Input: dimensioned drawing with shaded views. Units: mm. Origin: part minimum x, y, z. A direction names the side the tool comes from. Round coordinates to 2 decimals unless told otherwise and drop trailing zeros. Loops run counter-clockwise (first coordinate to the right, second up) from the corner with the lowest first, then second, coordinate; pieces in that order, holes last. Notation, with made-up numbers: M 81.25,17.25 L 123.25,17.25 A23 cw 123.25,47.25 Z; hole C 57,22 d2. An arc over 180 degrees is marked long. Answer as a JSON object with one key per item and string values.
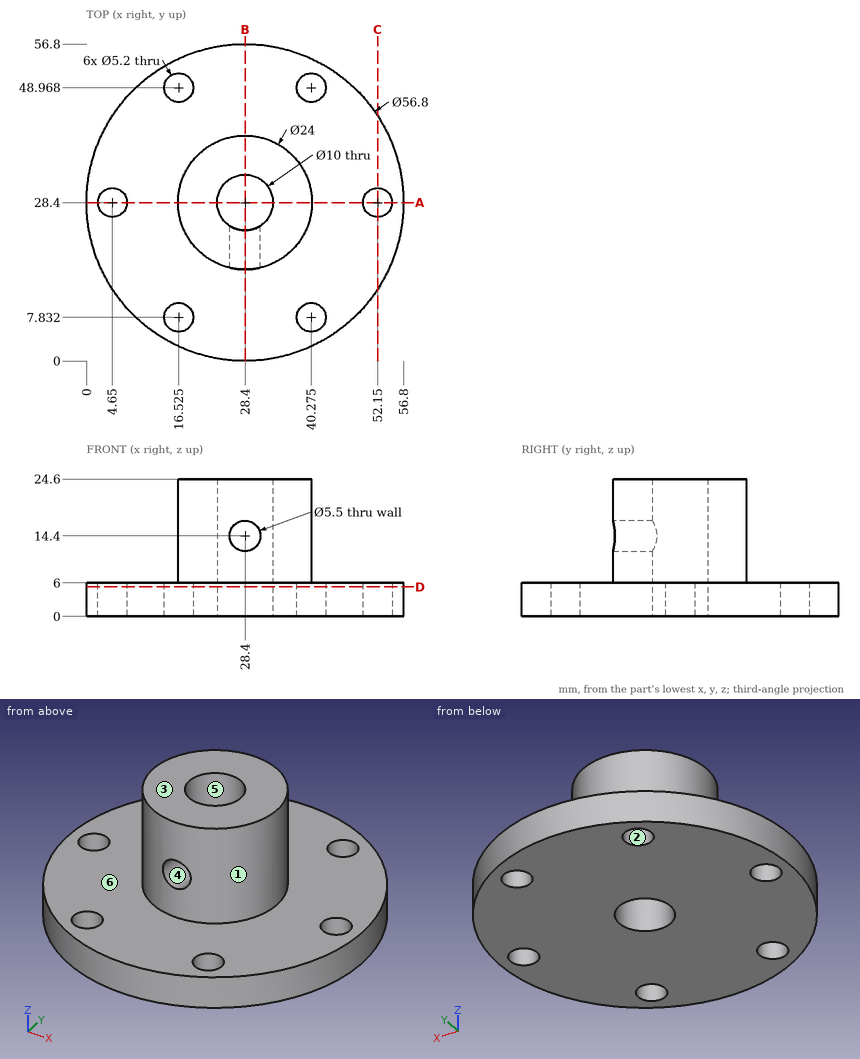
Item 1: Section D-D on z = 5.25. Return the cut outline in (x, y) (3 decimals).
Answer sheet:
{"outline": "C 28.4,28.4 d56.8; hole C 4.65,28.4 d5.2; hole C 16.525,7.832 d5.2; hole C 16.525,48.968 d5.2; hole C 28.4,28.4 d10; hole C 40.275,7.832 d5.2; hole C 40.275,48.968 d5.2; hole C 52.15,28.4 d5.2"}
Item 2: Section A-A on y = 28.4. Return the cut outline in (x, z), then the cut area to 3 significant figures.
Answer sheet:
{"outline": "M 0,0 L 2.05,0 L 2.05,6 L 0,6 Z; M 7.25,0 L 23.4,0 L 23.4,24.6 L 16.4,24.6 L 16.4,6 L 7.25,6 Z; M 33.4,0 L 49.55,0 L 49.55,6 L 40.4,6 L 40.4,24.6 L 33.4,24.6 Z; M 54.75,0 L 56.8,0 L 56.8,6 L 54.75,6 Z", "area": "479 mm²"}
Item 3: Access query for the marked faces 4, 5 and 6. Directions: +Z, -Z, +X, -X, +Y, -Y. A direction counts if a zero-diameter tool reaches every point of the face in a straight line with its end or side. Return the directions, or none.
Answer sheet:
{"face 4": "-Y", "face 5": "+Z, -Z", "face 6": "+Z"}
Item 4: Line query: probe 1 along Y at (x, z) = (40, 2.75); probe 2 along Z at (x, y) = (24.5, 43); probe 3 along X at (y, z) = (20, 14.4). Output: solid intervals per line, ascending. Write a range as from..to.
Answer sheet:
{"probe 1": "y = 2.48..5.25, 10.42..46.38, 51.55..54.32", "probe 2": "z = 0..6", "probe 3": "x = 19.83..25.65, 31.15..36.97"}
Item 5: Pull-direction query (X, two-part tool) for the marked faces 1, 2 and 3; classes: pulls with the +X half, pulls with the -X half, needs draft (parallel to the pull), parting line crosses it, or undercut.
Answer sheet:
{"face 1": "parting line crosses it", "face 2": "undercut", "face 3": "needs draft"}
Item 6: Section C-C on x = 52.15. Return the cut outline in (y, z), then the cut area to 3 significant figures.
Answer sheet:
{"outline": "M 12.83,0 L 25.8,0 L 25.8,6 L 12.83,6 Z; M 31,0 L 43.97,0 L 43.97,6 L 31,6 Z", "area": "156 mm²"}
Item 7: Section B-B on x = 28.4. Return the cut outline in (y, z).
Answer sheet:
{"outline": "M 0,0 L 23.4,0 L 23.4,11.65 L 16.4,11.65 L 16.4,6 L 0,6 Z; M 16.4,17.15 L 23.4,17.15 L 23.4,24.6 L 16.4,24.6 Z; M 33.4,0 L 56.8,0 L 56.8,6 L 40.4,6 L 40.4,24.6 L 33.4,24.6 Z"}
Item 8: Contact query for flat-ended pins moving along their axis: pin 1 Ø4 at (y, z) = (6.5, 3.5) entering from -X; pin 2 Ø4.5 at (x, z) = (28.4, 14.4) entering from -Y (3 decimals); pin 3 Ø3 at (x, y) = (52.15, 28.4) entering from -Z; pin 4 Ø8.5 at (x, y) = (16.52, 48.97) entering from -Z. Output: stop coordinate, or through.
Answer sheet:
{"pin 1": "stops at x = 8.14", "pin 2": "stops at y = 32.865", "pin 3": "passes through", "pin 4": "stops at z = 0"}
